from build123d import *

# Parameters (mm, degrees)
SKETCH1_R      = 5.5
SKETCH1_R_2    = 3.4
EXTRUDE1_DEPTH = 2
EXTRUDE2_START = 12
SKETCH2_R      = 5.5
EXTRUDE2_DEPTH = 12
SKETCH3_R      = 7
EXTRUDE3_DEPTH = 2


with BuildPart() as part:
    # Sketch1 → Extrude1 (new body)
    with BuildSketch(Plane.XY):
        Circle(SKETCH1_R)
        Circle(SKETCH1_R_2, mode=Mode.SUBTRACT)
    extrude(amount=EXTRUDE1_DEPTH)

    # Sketch2 → Extrude2 (add)
    with BuildSketch(Plane(origin=(0, 0, 0), x_dir=(-1, 0, 0), z_dir=(0, 0, -1)).offset(EXTRUDE2_START)):
        Circle(SKETCH2_R)
    extrude(amount=-EXTRUDE2_DEPTH)

    # Sketch3 → Extrude3 (add)
    with BuildSketch(Plane(origin=(0, 0, -12), x_dir=(-1, 0, 0), z_dir=(0, 0, -1))):
        Circle(SKETCH3_R)
    extrude(amount=EXTRUDE3_DEPTH)


solid = part.part
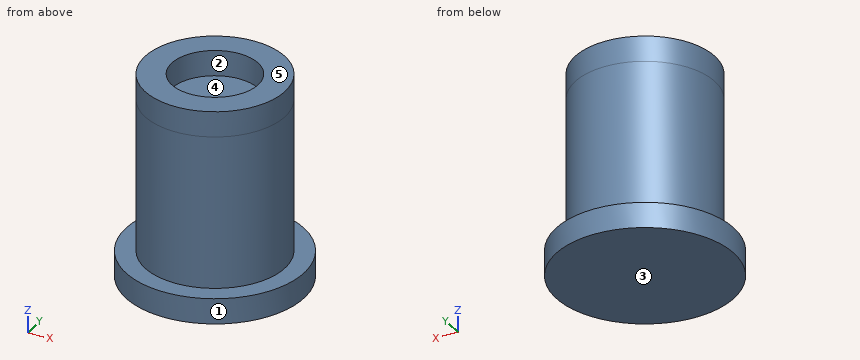
Design review of the part built by this model. Coordinates are the model's own, in mm. Face numbers are marked on the shaded views. A direction names the side the tool comes from. Round coordinates to 2 decimals unless told otherwise and drop trailing zeros. Loops run counter-clockwise (first coordinate to the right, second up) from the corner with the lowest first, then second, coordinate; pieces in that order, holes last. Notation, with made-up numbers: (58, -25) -> (102, -25) arc R15 ccw to (102, -20) -> close; hole circle Ø7 at (39.5, -19). An arc over 180 degrees is marked (long way). Use one line per item in the form item = value. Start each with the question number.
Q1. We need section D-D on x = 3.75. Give the boundary of the cut face in (y, z), then the cut area to 3 significant figures.
Q2. Wall thickness on line 1 along Y through (x, z) = (0, 0.8); line 2 along Z through (x, y) = (-0.25, 2.25); line 3 along Z through (x, y) = (-6, -2.25): over which ranges is each line inside the solid? List them lowest first. Write a range as [from, to].
Q3. Machinability: for the marked faces 4 and 5, which of the approach directions +Z, -Z, +X, -X, +Y, -Y give a long, thin tool a straight path to every point of the face, cutting with its end or side? Answer none if there is none.
Q4. For pin 1 Ø1 at (x, z) = (-4, -9.5) entering from -Y; pin 2 Ø2 at (y, z) = (1, -4.5) entering from +X; pin 3 Ø2 at (x, y) = (0, -1) entering from +Z, all flat-tipped, find the tip position at first contact; note any pin that passes through.
Q5. Draft analysis for pull direction X (two halves, no side actions). For the marked faces 1, 2 and 3, state which applies: +X half, -X half, draft (parallel to the pull), parting line (faces both ways), or undercut.
Q6. We need section C-C on z = -11. Give the boundary of the cut face in (x, y).
Q7. We need section A-A on x = 0. Give the boundary of the cut face in (y, z), then the cut area to 3 significant figures.
Calculated:
q1.outline = (-5.91, -14) -> (5.91, -14) -> (5.91, -12) -> (4.02, -12) -> (4.02, 2) -> (-4.02, 2) -> (-4.02, -12) -> (-5.91, -12) -> close
q1.area = 136 mm²
q2.line_1 = [-5.5, -3.4], [3.4, 5.5]
q2.line_2 = [-14, 0]
q2.line_3 = [-14, -12]
q3.face_4 = +Z
q3.face_5 = +Z, +X, -X, +Y, -Y
q4.pin_1 = -4.24
q4.pin_2 = 5.5
q4.pin_3 = 0
q5.face_1 = parting line
q5.face_2 = undercut
q5.face_3 = draft
q6.outline = circle Ø11 at (0, 0)
q7.outline = (-7, -14) -> (7, -14) -> (7, -12) -> (5.5, -12) -> (5.5, 2) -> (3.4, 2) -> (3.4, 0) -> (-3.4, 0) -> (-3.4, 2) -> (-5.5, 2) -> (-5.5, -12) -> (-7, -12) -> close
q7.area = 168 mm²
